```python
from build123d import *

# Parameters (mm, degrees)
BOSS_EXTRUDE1_DEPTH     = 2
EDGE_FLANGE1_DEPTH      = 2
EDGE_FLANGE1_BEND_DEPTH = 2
MOVE_FACE1_BY           = 5
CUT_EXTRUDE1_DEPTH      = 10


# Sheet-metal steps are written as plain solids
with BuildPart() as part:
    # Sketch1 → Boss-Extrude1 (new body)
    with BuildSketch(Plane(origin=(0, 0, 0), x_dir=(1, 0, 0), z_dir=(0, 1, 0))):
        Polygon((48.786990623, -23.171897133), (48.786990623, -13.328634875), (47.986992223, -12.528636475), (47.986992223, -9.428635055), (41.786991923, -3.228634755), (-54.913007717, -3.228634755), (-66.471417942, -3.228634755), (-66.471417942, -1.378635375), (-68.471417942, -1.378635375), (-68.471417942, 0.621364625), (-66.471417942, 0.621364625), (-66.471417942, 2.471364005), (-54.913007717, 2.471364005), (65.786992183, 2.471364005), (65.786992183, -1.128636415), (52.786992783, -1.128636415), (52.786992783, -11.528635935), (54.986990923, -13.728634075), (54.986993463, -14.428635215), (56.686992603, -16.128634355), (56.686992603, -42.528634895), (53.786993323, -45.428634175), (43.086991863, -45.428634175), (43.086991863, -34.028634115), (49.286992163, -34.028634115), (50.586992103, -32.728634175), (50.586992103, -30.828635435), (48.786990623, -29.028636495), (48.786990623, -25.171897133), (46.786990623, -25.171897133), (46.786990623, -23.171897133), align=None)
    extrude(amount=BOSS_EXTRUDE1_DEPTH)

    # Edge-Flange1 section (across the edge) → Edge-Flange1 (add)
    with BuildSketch(Plane(origin=(-69.471417942, 0, 1.378635375), x_dir=(1, 0, 0), z_dir=(0, 0, -1))):
        with BuildLine():
            Line((-2, 0.5), (-2, 1.4))
            Line((-2, 1.4), (0, 1.4))
            Line((0, 1.4), (0, 0.5))
            ThreePointArc((0, 0.5), (0.146446609, 0.146446609), (0.5, 0))
            Line((0.5, 0), (1, 0))
            Line((1, 0), (1, -2))
            Line((1, -2), (0.5, -2))
            ThreePointArc((0.5, -2), (-1.267766953, -1.267766953), (-2, 0.5))
        make_face()
    extrude(amount=EDGE_FLANGE1_DEPTH)

    # Edge-Flange1 section 2 (across the edge) → Edge-Flange1 bend (add)
    with BuildSketch(Plane(origin=(45.786990623, 0, 25.171897133), x_dir=(1, 0, 0), z_dir=(0, 0, -1))):
        with BuildLine():
            Line((-2, 0.5), (-2, 1.4))
            Line((-2, 1.4), (0, 1.4))
            Line((0, 1.4), (0, 0.5))
            ThreePointArc((0, 0.5), (0.146446609, 0.146446609), (0.5, 0))
            Line((0.5, 0), (1, 0))
            Line((1, 0), (1, -2))
            Line((1, -2), (0.5, -2))
            ThreePointArc((0.5, -2), (-1.267766953, -1.267766953), (-2, 0.5))
        make_face()
    extrude(amount=EDGE_FLANGE1_BEND_DEPTH)

    # Move Face1: a face moved outward by 5.0
    extrude(part.faces().sort_by_distance((65.786992183, 1, -0.671363795))[0], amount=MOVE_FACE1_BY, dir=(1, 0, 0))

    # Sketch12 → Cut-Extrude1 (cut)
    with BuildSketch(Plane(origin=(0, 2, 0), x_dir=(1, 0, 0), z_dir=(0, 1, 0))):
        Polygon((-52.913012042, -1.628639718), (-55.913012042, -1.628639718), (-55.913012042, -3.128639258), (-67.564249917, -3.128639258), (-67.671952829, -4.327104706), (41.886988858, -5.326407077), (48.086989158, -13.828640718), (48.007739716, -22.517187069), (46.286990623, -23.171897133), (48.886987558, -23.171897133), (48.886987558, -13.328639178), (48.086989158, -12.528640778), (48.086989158, -9.328639558), (41.886988858, -3.128639258), (31.786988738, -3.128639258), (31.786988738, -1.628639718), (28.886989458, -1.628639718), (28.886989458, -3.128639258), (15.186988918, -3.128639258), (15.186988918, -1.628639718), (12.286989638, -1.628639718), (12.286989638, -3.128639258), (-1.913012442, -3.128639258), (-1.913012442, -1.628639718), (-4.813011722, -1.628639718), (-4.813011722, -3.128639258), (-18.813011662, -3.128639258), (-18.813011662, -1.628639718), (-21.713010942, -1.628639718), (-21.713010942, -3.128639258), (-36.313012222, -3.128639258), (-36.313012222, -1.628639718), (-39.313011302, -1.628639718), (-39.313011302, -3.128639258), (-52.913012042, -3.128639258), align=None)
        Polygon((48.886987558, -25.171897133), (46.286990623, -25.171897133), (41.570815933, -34.028638418), (41.570815933, -47.167587605), (56.254650903, -46.954291818), (57.278434149, -42.02008581), (58.126913923, -16.761088184), (54.30540669, -8.580570975), (54.30540669, -2.3223377), (71.613193797, -2.589733287), (71.946410025, 3.760976012), (44.354427072, 3.760976012), (-68.474759816, 3.760976012), (-68.386329283, 2.371359902), (67.886988718, 2.371359902), (67.886988718, -1.028638378), (66.086988718, -1.028638378), (66.086988718, -0.128640178), (63.186989438, -0.128640178), (63.186989438, -1.028638378), (52.686987578, -1.028638378), (52.686987578, -1.528639918), (51.186988038, -1.528639918), (51.186988038, -4.228639598), (52.686987578, -4.228639598), (52.686987578, -11.528640238), (54.986988058, -13.828640718), (54.986988058, -14.528639318), (56.586989938, -16.128641198), (56.586989938, -42.428636858), (55.486987058, -43.528639738), (43.186988798, -43.528639738), (43.186988798, -35.428640698), (49.286986758, -35.428640698), (50.686989038, -34.028638418), (50.686989038, -30.728637398), (48.886987558, -28.928638458), align=None)
    extrude(amount=-CUT_EXTRUDE1_DEPTH, mode=Mode.SUBTRACT)


solid = part.part
```
Could you check a few things on this model? Use its own coordinates, in mm. A direction names the side the tool comes from. Give positions to 0.01 mm unless a question says otherwise; leave off trailing zeros. Loops run counter-clockwise (first coordinate to the right, second up) from the corner with the lowest first, then second, coordinate; pieces in that order, holes last. Notation, with made-up numbers: (5.25, 35.25) - (50.25, 35.25) arc R20 cw to (50.25, 68.25) - close; hole circle Ø3 at (-23.5, -15.5). An arc over 180 degrees is marked (long way). Answer in a Markdown table with one row per item. Add a question column.
Q1. For pin 1 (1 mm diameter, centred on x = -55, y = 1, fed in from +Z); pin 2 (0.6 mm diameter, centred on y = 0.5, z = 32.5, fed in from +X); pin 3 (0.6 mm diameter, centred on x = 8, y = 1, fed in from +Z), each with a flat end and sliding along its axis, tell me the tip position at first contact or that it passes through.
Q2. If we section it at A-A (x = 37): List the corners of the cut face in (y, z) for me.
Q3. Which directions (+Z, -Z, +X, -X, +Y, -Y) give clear straight access to the entire face, cutting with the end or side of a thin tool? Please do faces 1 (the face through (-69, 1, 1.379)), 2 (the face through (46, 1, 25.172)), 3 (the face through (-69, 1, -0.621)), 4 (the face through (44.54, 1.29, 24.19)).
Q4. If we section it at B-B (z = 21.5): List the corners of the cut face in (x, y) for me, plus the area to 3 significant figures.
Q5. Please list where these lines run through material, in increasing order: L1, parallel to Z at x = 51.5, y = 0.4; L2, parallel to X at y = 1, z = 10; L3, parallel to Z at x = 0, y = 1.8. Write a range as from..to.
The answers:
| question | item | result |
|---|---|---|
| 1 | pin 1 | stops at z = 1.63 |
| 1 | pin 2 | stops at x = 56.59 |
| 1 | pin 3 | stops at z = 3.13 |
| 2 | outline | (0, -2.37) - (2, -2.37) - (2, 3.13) - (0, 3.13) - close |
| 3 | face 1 | +Z, -X, +Y, -Y |
| 3 | face 2 | -X, +Y, -Y |
| 3 | face 3 | -Z, -X, +Y, -Y |
| 3 | face 4 | -X, +Y |
| 4 | outline | (48.89, 0) - (56.59, 0) - (56.59, 2) - (48.89, 2) - close |
| 4 | area | 15.4 mm^2 |
| 5 | L1 | z = -2.37..1.53, 4.23..43.53 |
| 5 | L2 | x = 48.09..52.69 |
| 5 | L3 | z = -2.37..3.13 |
